from build123d import *

# Parameters (mm, degrees)
F0_W     = 300
F0_H     = 300
F0_W_2   = 240
F0_H_2   = 240
F1_DEPTH = 30
F2_W     = 30
F2_H     = 30
F3_DEPTH = 240


with BuildPart() as f1:
    # F0 (on Top) → F1 (new body)
    with BuildSketch(Plane.XY):
        Rectangle(F0_W, F0_H)
        Rectangle(F0_W_2, F0_H_2, mode=Mode.SUBTRACT)
    extrude(amount=F1_DEPTH)

    # F2 (on face) → F3 (join)
    with BuildSketch(Plane.XY.offset(30)):
        with Locations((-135, 135)):
            Rectangle(F2_W, F2_H)
        with Locations((135, 135)):
            Rectangle(F2_W, F2_H)
        with Locations((135, -135)):
            Rectangle(F2_W, F2_H)
        with Locations((-135, -135)):
            Rectangle(F2_W, F2_H)
    extrude(amount=F3_DEPTH)


solid = f1.part
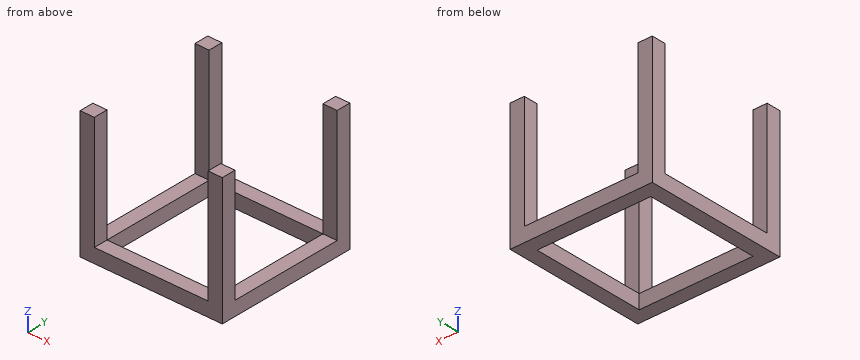
The listing builds one solid part. Answer for the finished solid, in the listing's coordinates (mm). Give positions to 0.01 mm unless a question says otherwise; leave off trailing zeros. Loops run counter-clockwise (first coordinate to the right, second up) from the corner with the lowest first, then second, coordinate; pieces in that order, holes last. Notation, with made-up numbers: (63.25, 26) - (82.25, 26) arc R21 cw to (82.25, 34) - close; hole circle Ø8 at (0.25, 84.25). An arc over 180 degrees is marked (long way). Answer as a JSON object with one key per item and string values.
1. A cutting plane is placed at B-B (y = 60.5). Write down the section's boundary in (x, z).
Determined:
{"outline": "(-150, 0) - (-120, 0) - (-120, 30) - (-150, 30) - close; (120, 0) - (150, 0) - (150, 30) - (120, 30) - close"}
2. A cutting plane is placed at D-D (x = -130). Write down the section's boundary in (y, z), then the cut area to 3 significant figures.
Determined:
{"outline": "(-150, 0) - (150, 0) - (150, 270) - (120, 270) - (120, 30) - (-120, 30) - (-120, 270) - (-150, 270) - close", "area": "23,400 mm²"}
3. A cutting plane is placed at A-A (z = 187.5). Write down the section's boundary in (x, y).
Determined:
{"outline": "(-150, -150) - (-120, -150) - (-120, -120) - (-150, -120) - close; (-150, 120) - (-120, 120) - (-120, 150) - (-150, 150) - close; (120, -150) - (150, -150) - (150, -120) - (120, -120) - close; (120, 120) - (150, 120) - (150, 150) - (120, 150) - close"}
4. Find the intervals of material crossed by L1, parallel to Y at x = 134.5, z = 91; L2, parallel to Z at x = -132, y = -110, in increasing order. Write a range as [from, to].
Determined:
{"L1": "[-150, -120], [120, 150]", "L2": "[0, 30]"}
5. A flat-ended cylindrical pin translates along its axis: pin 1 Ø15 at (x, y) = (56.5, -130.5) entering from +Z. Find the tip coordinate at first contact, or state that the pin passes through.
Determined:
{"pin 1": "z = 30"}
